Source: CAD feature listing. Evaluate the final solid. Frame: model axes, mm. Face numbers are marked on the shaded views. A direction names the side the tool comes from. Coordinates: 2 decimals unless noted, no trailing zeros. Loops run counter-clockwise (first coordinate to the right, second up) from the corner with the lowest first, then second, coordinate; pieces in that order, holes last.
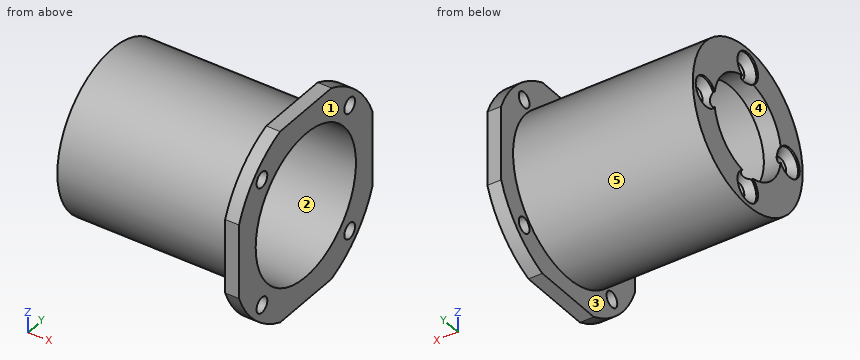
```python
from build123d import *

# Parameters (mm, degrees)
HOLE_WIZARD_2_AT_2_COUNT = 2
HOLE_WIZARD_2_AT_2_PITCH = 24.748737342
HOLE_WIZARD_2_AT_3_COUNT = 2
HOLE_WIZARD_2_AT_3_PITCH = 35
HOLE_WIZARD_2_AT_4_COUNT = 2
HOLE_WIZARD_2_AT_4_PITCH = 24.748737342
SKETCH_18_OUTSIDE_W      = 82.334
SKETCH_18_OUTSIDE_H      = 82.334
SKETCH_18_OUTSIDE_W_2    = 56
SKETCH_18_OUTSIDE_H_2    = 56
CUT_EXTRUDE_3_DEPTH      = 4
HOLE_WIZARD_M4_1_D       = 4.5


with BuildPart() as part:
    # 草图1 → 旋转2 (revolve)
    with BuildSketch(Plane.XY, mode=Mode.PRIVATE) as revolve_2_sk:
        Polygon((52, 23), (52, 30), (56, 30), (56, 21), (5, 21), (5, 14), (0, 14), (0, 23), align=None)
    revolve(revolve_2_sk.sketch.rotate(Axis((0, 0, 0), (1, 0, 0)), 180), axis=Axis((0, 0, 0), (1, 0, 0)))

    # 草图10 → 打孔尺寸根据十字槽沉头木螺钉的类型2 (revolve, cut)
    with BuildSketch(Plane(origin=(0, 0, 17.5), x_dir=(0, 0, 1), z_dir=(0, 1, 0))):
        Polygon((0, 0), (0, 56), (2.25, 56), (2.25, 2.55), (4.3, 0.5), (4.3, 0), align=None)
    hole_wizard_2 = revolve(axis=Axis((-6.35, 0, 17.5), (1, 0, 0)), mode=Mode.SUBTRACT)

    # 打孔尺寸根据十字槽沉头木螺钉的类型2 at 2: 打孔尺寸根据十字槽沉头木螺钉的类型2 ×2
    with Locations(*[Vector(0, -0.7071067811865575, -0.7071067811865376) * (i * HOLE_WIZARD_2_AT_2_PITCH) for i in range(1, HOLE_WIZARD_2_AT_2_COUNT)]):
        add(hole_wizard_2, mode=Mode.SUBTRACT)

    # 打孔尺寸根据十字槽沉头木螺钉的类型2 at 3: 打孔尺寸根据十字槽沉头木螺钉的类型2 ×2
    with Locations(*[(0, 0, -i * HOLE_WIZARD_2_AT_3_PITCH) for i in range(1, HOLE_WIZARD_2_AT_3_COUNT)]):
        add(hole_wizard_2, mode=Mode.SUBTRACT)

    # 打孔尺寸根据十字槽沉头木螺钉的类型2 at 4: 打孔尺寸根据十字槽沉头木螺钉的类型2 ×2
    with Locations(*[Vector(0, 0.7071067811865376, -0.7071067811865575) * (i * HOLE_WIZARD_2_AT_4_PITCH) for i in range(1, HOLE_WIZARD_2_AT_4_COUNT)]):
        add(hole_wizard_2, mode=Mode.SUBTRACT)

    # 草图18 outside → 切除-拉伸3 (cut)
    with BuildSketch(Plane(origin=(56, 0, 0), x_dir=(0, 0, -1), z_dir=(1, 0, 0))):
        Rectangle(SKETCH_18_OUTSIDE_W, SKETCH_18_OUTSIDE_H)
        Rectangle(SKETCH_18_OUTSIDE_W_2, SKETCH_18_OUTSIDE_H_2, mode=Mode.SUBTRACT)
    extrude(amount=-CUT_EXTRUDE_3_DEPTH, mode=Mode.SUBTRACT)

    # M4 间隙孔1 (through all)
    with Locations(Plane(origin=(56, 0, 0), x_dir=(0, 0, -1), z_dir=(1, 0, 0))):
        with Locations((18.384776311, 18.384776311), (18.384776311, -18.384776311), (-18.384776311, -18.384776311), (-18.384776311, 18.384776311)):
            Hole(HOLE_WIZARD_M4_1_D / 2)


solid = part.part
```
Q1. Section query D-D on x = 4. Return the cut outline in (y, z).
Q2. Draft query along Y for the marked faces 3, 4 and 5. Return one class per face: released by +Y, released by -Y, zero draft, split by the parting line, or undercut.
Q3. Reachability of the marked faces 1 and 2 from +Z, -Z, +X, -X, +Y, -Y: full face, straight path, thin tool, end or side. Return the list, or none.
Q4. Section query C-C on y = 7.5. Return the cut outline in (x, z), then the cut area to 3 significant figures.
Q5. First-contact query: pin 1 Ø5 at (y, z) = (0, 17.5) entering from -X; pin 2 Ø7 at (y, z) = (-17.5, 0) entering from -X; pin 3 Ø5 at (y, z) = (12, 7.5) entering from +X. Flat tips, straight axial feed; report the tip coordinate or a pass-through.
Q6. Material intervals for line 1 along Z through (x, y) = (2.9, 0); line 2 along X through (y, z) = (15, -7.5); line 3 along Z through (x, y) = (25.5, -9.5), sorted ascending.
Q7. Section query A-A on z = 0. Return the cut outline in (x, y), then the cut area to 3 significant figures.
Resolved:
1. outline: circle Ø46 at (0, 0); hole circle Ø4.5 at (-17.5, 0); hole circle Ø28 at (0, 0); hole circle Ø4.5 at (0, -17.5); hole circle Ø4.5 at (0, 17.5); hole circle Ø4.5 at (17.5, 0)
2. face 3: zero draft
2. face 4: undercut
2. face 5: split by the parting line
3. face 1: +Z, -Z, +X, +Y, -Y
3. face 2: +X
4. outline: (0, -21.74) - (52, -21.74) - (52, -28) - (56, -28) - (56, -19.62) - (5, -19.62) - (5, -11.82) - (0, -11.82) - close; (0, 11.82) - (5, 11.82) - (5, 19.62) - (56, 19.62) - (56, 28) - (52, 28) - (52, 21.74) - (0, 21.74) - close
4. area: 366 mm2
5. pin 1: stops at x = 2.3
5. pin 2: stops at x = 1.3
5. pin 3: stops at x = 5
6. line 1: z = -23 to -19.75, -15.25 to -14, 14 to 15.25, 19.75 to 23
6. line 2: x = 0 to 5
6. line 3: z = -20.95 to -18.73, 18.73 to 20.95
7. outline: (0, -23) - (52, -23) - (52, -28) - (56, -28) - (56, -21) - (5, -21) - (5, -19.75) - (2.55, -19.75) - (0.5, -21.8) - (0, -21.8) - close; (0, 21.8) - (0.5, 21.8) - (2.55, 19.75) - (5, 19.75) - (5, 21) - (56, 21) - (56, 28) - (52, 28) - (52, 23) - (0, 23) - close; (1.3, -14) - (2.55, -15.25) - (5, -15.25) - (5, -14) - close; (1.3, 14) - (5, 14) - (5, 15.25) - (2.55, 15.25) - close
7. area: 278 mm2
